Read the model definition and answer for the solid it produces. Units are mm, in the model's axes. A direction names the side the tool comes from. Give positions to 0.01 mm unless a question says otherwise; leave off trailing zeros. Order: outer loops, then holes, each group sorted by start corner. A loop starts at its lowest first (then second) coordinate and runs counter-clockwise, first axis right, second up. Notation, with made-up numbers: (82.5, 69) - (138.5, 69) arc R22 cw to (138.5, 99) - close; hole circle Ø8 at (-28, -39.75). An arc over 180 degrees is marked (long way). Return JSON: item names as keys, results as strings.
```python
from build123d import *

# Parameters (mm, degrees)
F0_W     = 139.7
F0_H     = 88.9
F1_DEPTH = 76.2


with BuildPart() as f1:
    # F0 (on Front) → F1 (new body, symmetric)
    with BuildSketch(Plane.XZ):
        with BuildLine():
            Line((69.85, 50.8), (-69.85, 50.8))
            ThreePointArc((-69.85, 50.8), (-74.340128, 48.940128), (-76.2, 44.45))
            Line((-76.2, 44.45), (-76.2, -44.45))
            ThreePointArc((-76.2, -44.45), (-74.340128, -48.940128), (-69.85, -50.8))
            Line((-69.85, -50.8), (69.85, -50.8))
            ThreePointArc((69.85, -50.8), (74.340128, -48.940128), (76.2, -44.45))
            Line((76.2, -44.45), (76.2, 44.45))
            ThreePointArc((76.2, 44.45), (74.340128, 48.940128), (69.85, 50.8))
        make_face()
        Rectangle(F0_W, F0_H, mode=Mode.SUBTRACT)
    extrude(amount=F1_DEPTH, both=True)


solid = f1.part
```
Q1. Determine the mould class of faces 1 (the flat face through (1, -1, 50.8)), 2 (the flat face through (-1, -1, 44.45)), 3 (the flat face through (-6, 76.2, -45)) for opening direction Z: released by +Z, released by -Z, zero draft, split by the parting line, or undercut.
Values:
{"face 1": "released by +Z", "face 2": "undercut", "face 3": "zero draft"}
Q2. Consider L1, parallel to X at y = -27, z = -36.5; L2, parallel to Z at x = -32, y = 43.5; L3, parallel to X at y = 44, z = 45. Determine where each line is inside the solid, lowest interval first.
Values:
{"L1": "x = -76.2 to -69.85, 69.85 to 76.2", "L2": "z = -50.8 to -44.45, 44.45 to 50.8", "L3": "x = -76.18 to 76.18"}
Q3. A cutting plane is placed at C-C (z = -2.5). Write down the section's boundary in (x, y).
Values:
{"outline": "(-76.2, -76.2) - (-69.85, -76.2) - (-69.85, 76.2) - (-76.2, 76.2) - close; (69.85, -76.2) - (76.2, -76.2) - (76.2, 76.2) - (69.85, 76.2) - close"}
Q4. A cutting plane is placed at A-A (x = 55). Write down the section's boundary in (y, z).
Values:
{"outline": "(-76.2, -50.8) - (76.2, -50.8) - (76.2, -44.45) - (-76.2, -44.45) - close; (-76.2, 44.45) - (76.2, 44.45) - (76.2, 50.8) - (-76.2, 50.8) - close"}
Q5. A cutting plane is placed at B-B (y = -61.5). Write down the section's boundary in (x, z), and give its area (3 significant figures).
Values:
{"outline": "(-76.2, -44.45) arc R6.35 ccw to (-69.85, -50.8) - (69.85, -50.8) arc R6.35 ccw to (76.2, -44.45) - (76.2, 44.45) arc R6.35 ccw to (69.85, 50.8) - (-69.85, 50.8) arc R6.35 ccw to (-76.2, 44.45) - close; hole (-69.85, -44.45) - (69.85, -44.45) - (69.85, 44.45) - (-69.85, 44.45) - close", "area": "3,030 mm²"}
Q6. For faces 4 (the cylindrical face through (74.29, -1.07, -48.99)), 5 (the flat face through (69.85, -1, -1)), determine the directions among +Z, -Z, +X, -X, +Y, -Y from which every point of the face is accessible in a straight line to the end or side of a thin tool.
Values:
{"face 4": "-Z, +X, +Y, -Y", "face 5": "+Y, -Y"}
